from build123d import *

# Parameters (mm, degrees)
SKETCH2_R          = 0.79375
CUT_EXTRUDE1_DEPTH = 13.61848379


with BuildPart() as part:
    # Sketch1 → Revolve1 (revolve)
    with BuildSketch(Plane(origin=(0, 0, 0), x_dir=(1, 0, 0), z_dir=(0, 1, 0)), mode=Mode.PRIVATE) as revolve1_sk:
        with BuildLine():
            Line((-8.8646, 3.175), (0, 3.175))
            Line((0, 3.175), (0, 4.630987194))
            Line((0, 4.630987194), (-0.449012806, 5.08))
            Line((-0.449012806, 5.08), (-4.445, 5.08))
            Line((-4.445, 5.08), (-4.445, 6.35))
            Line((-4.445, 6.35), (-5.715, 6.35))
            ThreePointArc((-5.715, 6.35), (-6.6548, 5.4102), (-7.5946, 6.35))
            Line((-7.5946, 6.35), (-8.8646, 6.35))
            Line((-8.8646, 6.35), (-8.8646, 3.175))
        make_face()
    revolve(revolve1_sk.sketch.rotate(Axis((-10.922, 0, 0), (1, 0, 0)), 180), axis=Axis((-10.922, 0, 0), (1, 0, 0)))

    # Sketch2 → Cut-Extrude1 (cut, through all)
    with BuildSketch(Plane(origin=(0, 0, 0), x_dir=(1, 0, 0), z_dir=(0, 1, 0))):
        with Locations(Location((-2.427185556, 0, 0), (0, 0, 90))):
            Circle(SKETCH2_R)
    extrude(amount=CUT_EXTRUDE1_DEPTH, mode=Mode.SUBTRACT)


solid = part.part
Read the model definition and answer for the solid it produces. Units are mm, in the model's axes. A direction names the side the tool comes from. Give positions to 0.01 mm unless a question says otherwise; leave off trailing zeros. Write each loop counter-clockwise with the first axis right and the second up, starting at its lowest first coordinate (ties: lowest second). Pieces come first, ordered by that corner, then holes. Notation, with made-up numbers: M 66.5,56 L 77.5,56 A18 cw 77.5,82 Z; hole C 3,46 d4. An arc over 180 degrees is marked long. One line per item, written item: value. Start each with the question number.
(1) A tool of negligible diameter and unlimited length cuts with its end or side. For faces 1 (the cylindrical face through (-1.723, 4.064, -0.366)), 2 (the flat face through (-4.445, -5, -2)), 3 (the cylindrical face through (-8.238, 5.634, 2.93)), from which of +Z, -Z, +X, -X, +Y, -Y can it reach the whole face along a straight path? Write none if from no direction.
(2) Find section A-A (z = 0). Determine the outline of the cut face in (x, y) (3 decimals).
(3) Determine the mould class of faces 4 (the cylindrical face through (-4.37, -3.15, -0.41)), 5 (the flat face through (0, -3.2, -1)), 6 (the cylindrical face through (-5.089, 5.634, 2.93)) for opening direction Z: pulls with the +Z half, pulls with the -Z half, needs draft (parallel to the pull), parting line crosses it, or undercut.
(4) Find the intervals of material crossed by line 1 (Y direction, x = -4.75, z = 0) (3 decimals); line 2 (X direction, y = 3.65, z = 0); line 3 (Y direction, x = -4.5, z = 2.25), in increasing order.
(5) Find section C-C (x = -1). Determine the outline of the cut face in (y, z) (3 decimals).
(6) Find section B-B (x = -5). Determine the outline of the cut face in (y, z) (3 decimals).
(7) Flat-ended cylindrical pins translate along their axes: pin 1 Ø5 at (x, y) = (-1.5, -3) entering from -Z; pin 2 Ø1 at (y, z) = (1, -0.5) entering from +X; pin 3 Ø2 at (x, z) = (-8, 4.5) entering from +Y; pin 4 Ø2.5 at (x, z) = (-2.43, 0) entering from +Y. Find the tip coordinate at first contact, or state that the pin passes through.
Results below:
1. face 1: +Y
1. face 2: +X
1. face 3: +X, -X
2. outline: M -8.865,-6.35 L -7.595,-6.35 A0.94 cw -5.715,-6.35 L -4.445,-6.35 L -4.445,-5.08 L -0.449,-5.08 L 0,-4.631 L 0,-3.175 L -8.865,-3.175 Z; M -8.865,3.175 L -3.221,3.175 L -3.221,5.08 L -4.445,5.08 L -4.445,6.35 L -5.715,6.35 A0.94 cw -7.595,6.35 L -8.865,6.35 Z; M -1.633,3.175 L 0,3.175 L 0,4.631 L -0.449,5.08 L -1.633,5.08 Z
3. face 4: undercut
3. face 5: needs draft
3. face 6: parting line crosses it
4. line 1: y = -6.35 to -3.175, 3.175 to 6.35
4. line 2: x = -8.86 to -3.22, -1.63 to 0
4. line 3: y = -5.94 to -2.24, 2.24 to 5.94
5. outline: C 0,0 d10.16; hole C 0,0 d6.35
6. outline: C 0,0 d12.7; hole C 0,0 d6.35
7. pin 1: stops at z = -5.06
7. pin 2: passes through
7. pin 3: stops at y = 5.3
7. pin 4: stops at y = 5.08
